Here's how the part is built. I have some questions about the finished solid (model axes, mm). Face numbers are marked on the shaded views. A direction names the side the tool comes from. Round coordinates to 2 decimals unless told otherwise and drop trailing zeros. Loops run counter-clockwise (first coordinate to the right, second up) from the corner with the lowest first, then second, coordinate; pieces in that order, holes last. Notation, with made-up numbers: M -3.75,26 L 20.25,26 A17 ccw 20.25,43 Z; hole C 65,43.5 d8. An arc over 180 degrees is marked long. Use a Markdown table: item, result.
```python
from build123d import *

# Parameters (mm, degrees)
SKETCH_1_W          = 35
SKETCH_1_H          = 43.5
EXTRUDE_1_DEPTH     = 20
SKETCH_2_W          = 20
SKETCH_2_H          = 5
EXTRUDE_2_DEPTH     = 10
SKETCH_3_W          = 20
SKETCH_3_H          = 5
EXTRUDE_3_DEPTH     = 10
SKETCH_4_R          = 1.5
CUT_EXTRUDE_2_DEPTH = 5
SKETCH_5_R          = 12.25
CUT_EXTRUDE_3_DEPTH = 20


with BuildPart() as part:
    # Эскиз1 → Бобышка-Вытянуть1 (new body)
    with BuildSketch(Plane.XY):
        Rectangle(SKETCH_1_W, SKETCH_1_H)
    extrude(amount=EXTRUDE_1_DEPTH)

    # Эскиз2 → Бобышка-Вытянуть2 (add)
    with BuildSketch(Plane(origin=(17.5, 0, 0), x_dir=(0, 0, -1), z_dir=(1, 0, 0))):
        with Locations((-10, -19.25)):
            Rectangle(SKETCH_2_W, SKETCH_2_H)
    extrude(amount=EXTRUDE_2_DEPTH)

    # Эскиз3 → Бобышка-Вытянуть3 (add)
    with BuildSketch(Plane.ZY.offset(17.5)):
        with Locations((10, -19.25)):
            Rectangle(SKETCH_3_W, SKETCH_3_H)
    extrude(amount=EXTRUDE_3_DEPTH)

    # Эскиз4 → Вырез-Вытянуть2 (cut)
    with BuildSketch(Plane(origin=(0, -16.75, 0), x_dir=(1, 0, 0), z_dir=(0, 1, 0))):
        with Locations((-22.5, -16)):
            Circle(SKETCH_4_R)
        with Locations((-22.5, -4)):
            Circle(SKETCH_4_R)
        with Locations((22.5, -16)):
            Circle(SKETCH_4_R)
        with Locations((22.5, -4)):
            Circle(SKETCH_4_R)
    extrude(amount=-CUT_EXTRUDE_2_DEPTH, mode=Mode.SUBTRACT)

    # Эскиз5 → Вырез-Вытянуть3 (cut)
    with BuildSketch(Plane(origin=(0, 0, 0), x_dir=(-1, 0, 0), z_dir=(0, 0, -1))):
        with Locations((0, 8.25)):
            Circle(SKETCH_5_R)
    extrude(amount=-CUT_EXTRUDE_3_DEPTH, mode=Mode.SUBTRACT)


solid = part.part
```
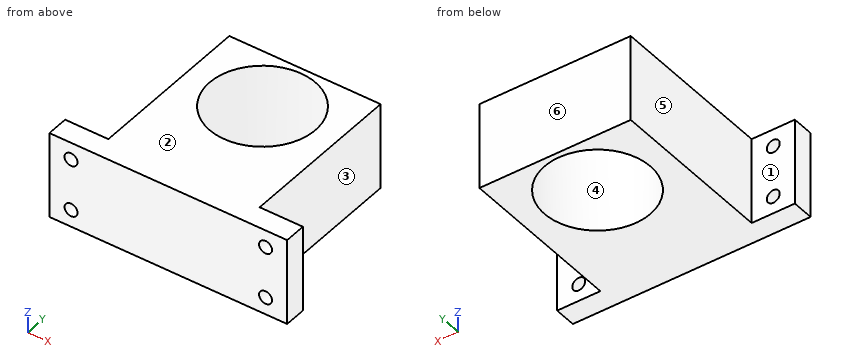
Q1. Imagine slicing it at B-B, the plane z = 4. Please give me the cut outline in (x, y).
Return value:
| item | result |
|---|---|
| outline | M -27.5,-21.75 L -24,-21.75 L -24,-16.75 L -27.5,-16.75 Z; M -21,-21.75 L 21,-21.75 L 21,-16.75 L 17.5,-16.75 L 17.5,21.75 L -17.5,21.75 L -17.5,-16.75 L -21,-16.75 Z; M 24,-21.75 L 27.5,-21.75 L 27.5,-16.75 L 24,-16.75 Z; hole C 0,8.25 d24.5 |
Q2. Imagine slicing it at D-D, the plane x = 4.5. Please give me the cut outline in (y, z), then the cut area to 3 significant figures.
Return value:
| item | result |
|---|---|
| outline | M -21.75,0 L -3.14,0 L -3.14,20 L -21.75,20 Z; M 19.64,0 L 21.75,0 L 21.75,20 L 19.64,20 Z |
| area | 414 mm^2 |
Q3. I need wall thicknesses on line 1 (X direction, y = -18.6, z = 16); line 2 (Z direction, x = -22.5, y = -19.85); line 3 (Z direction, x = 22, y = -19). Which ranges of each line are inside material? Lowest first, please. Write a range as from..to.
Return value:
| item | result |
|---|---|
| line 1 | x = -27.5..-24, -21..21, 24..27.5 |
| line 2 | z = 0..2.5, 5.5..14.5, 17.5..20 |
| line 3 | z = 0..2.59, 5.41..14.59, 17.41..20 |
Q4. For the marked faces 1, 2 and 3, which set-ups out of +Z, -Z, +X, -X, +Y, -Y let a thin tool reach every point of the face, with its end or its side?
Return value:
| item | result |
|---|---|
| face 1 | +Z, -Z, -X, +Y |
| face 2 | +Z, +X, -X, +Y, -Y |
| face 3 | +Z, -Z, +X, +Y |
Q5. We'd pull the mould along X, two halves only. Please class the marked faces 4, 5 and 6: pulls with the +X half, pulls with the -X half, needs draft (parallel to the pull), parting line crosses it, or undercut.
Return value:
| item | result |
|---|---|
| face 4 | undercut |
| face 5 | pulls with the -X half |
| face 6 | needs draft |
Q6. Imagine slicing it at C-C, the plane z = 11.5. Please give me the cut outline in (x, y), then the cut area to 3 significant figures.
Return value:
| item | result |
|---|---|
| outline | M -27.5,-21.75 L 27.5,-21.75 L 27.5,-16.75 L 17.5,-16.75 L 17.5,21.75 L -17.5,21.75 L -17.5,-16.75 L -27.5,-16.75 Z; hole C 0,8.25 d24.5 |
| area | 1,150 mm^2 |
Q7. Imagine slicing it at A-A, the plane x = 22.5. Please give me the cut outline in (y, z).
Return value:
| item | result |
|---|---|
| outline | M -21.75,0 L -16.75,0 L -16.75,2.5 L -21.75,2.5 Z; M -21.75,5.5 L -16.75,5.5 L -16.75,14.5 L -21.75,14.5 Z; M -21.75,17.5 L -16.75,17.5 L -16.75,20 L -21.75,20 Z |
Q8. Will these pins go through, and if not, where does the flat tip stop? P1, Ø4, axis at x = -22.5, z = 4, coming from the +Y side; P2, Ø4, axis at y = 0.5, z = 17.5, coming from the +X side; P3, Ø1, axis at y = -1, z = 12, coming from the -X side.
Return value:
| item | result |
|---|---|
| P1 | stops at y = -16.75 |
| P2 | stops at x = 17.5 |
| P3 | stops at x = -17.5 |
